Geometry: final body of the model. Coordinates: model frame, mm. Face numbers are marked on the shaded views. A direction names the side the tool comes from. Coordinates: 2 decimals unless noted, no trailing zeros. Write each loop counter-clockwise with the first axis right and the second up, starting at its lowest first coordinate (ties: lowest second). Pieces come first, ordered by that corner, then holes. Notation, with made-up numbers: (31.25, 79.5) -> (50.25, 79.5) arc R21 ccw to (50.25, 101.5) -> close; hole circle Ø10 at (48.5, 52). An arc over 180 degrees is marked (long way). One line per item, written item: value.
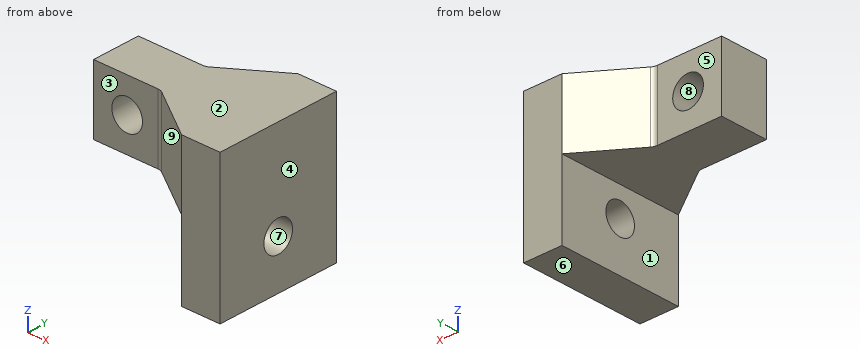
Autodesk Inventor part; units mm, degrees
ref_plane "YZ Plane" through (0, 0, 0) normal (1, 0, 0) x (0, 1, 0)
ref_plane "XZ Plane" through (0, 0, 0) normal (0, 1, 0) x (-1, 0, 0)
ref_plane "XY Plane" through (0, 0, 0) normal (0, 0, 1) x (1, 0, 0)
sketch "Sketch1" plane through (0, 0, 0) normal (1, 0, 0) x (0, 1, 0)
  circle A0 centre (0, 0) radius 1.6
  line L0 (0, 0) -> (0, -66.3)
  circle A1 centre (0, -66.3) radius 1.6
  line L1 (0, 0) -> (3.5, 0)
  line L2 (3.5, 0) -> (3.5, 3.5)
  line L3 (3.5, 3.5) -> (-3.5, 3.5)
  line L4 (-3.5, 3.5) -> (-3.5, -3.5)
  line L5 (-3.5, -3.5) -> (3.5, -3.5)
  line L6 (3.5, -3.5) -> (3.5, 0)
  line L7 (0, -66.3) -> (3.5, -66.3)
  line L8 (3.5, -66.3) -> (3.5, -62.8)
  line L9 (3.5, -62.8) -> (-3.5, -62.8)
  line L10 (-3.5, -62.8) -> (-3.5, -69.8)
  line L11 (-3.5, -69.8) -> (3.5, -69.8)
  line L12 (3.5, -69.8) -> (3.5, -66.3)
  line L13 (3.5, 3.5) -> (3.5, 6.5)
  line L14 (3.5, 6.5) -> (-3.5, 6.5)
  line L15 (-3.5, 6.5) -> (-3.5, 3.5)
  line L16 (3.5, -69.8) -> (3.5, -72.8)
  line L17 (3.5, -72.8) -> (-3.5, -72.8)
  line L18 (-3.5, -72.8) -> (-3.5, -69.8)
  dimension "d0" = 3.2
  dimension "d1" = 66.3
  dimension "d2" = 3.2
  dimension "d3" = 3.5
  dimension "d4" = 3.5
  dimension "d5" = 7
  dimension "d6" = 7
  dimension "d7" = 3.5
  dimension "d8" = 3.5
  dimension "d9" = 7
  dimension "d10" = 7
  dimension "d11" = 3
  dimension "d12" = 3
extrude "Extrusion1" add sketch "Sketch1" along normal blind 3 contours L1 L6 L5 L0 A0 | A0 L0 L5 L4 L3 L2 L1 | L9 L8 L7 A1 L0 | L0 A1 L7 L12 L11 L10 L9 | L3 L15 L14 L13 | L11 L16 L17 L18
sketch "Sketch2" plane through (3, 0, 0) normal (1, 0, 0) x (0, 0, -1)
  line L0 (-6.5, 3.5) -> (-6.5, -3.5)
  line L1 (-6.5, -3.5) -> (3.5, -3.5)
  line L2 (3.5, -3.5) -> (3.5, 3.5)
  line L3 (3.5, 3.5) -> (-6.5, 3.5)
  circle A0 centre (0, 0) radius 1.6
  line L4 (62.8, -3.5) -> (72.8, -3.5)
  line L5 (72.8, -3.5) -> (72.8, 3.5)
  line L6 (72.8, 3.5) -> (62.8, 3.5)
  line L7 (62.8, 3.5) -> (62.8, -3.5)
  circle A1 centre (66.3, 0) radius 1.6
  line L8 (-6.5, 3.5) -> (-6.5, -3.5)
  line L9 (-6.5, 3.5) -> (-2.5, 3.5)
  line L10 (3.5, 3.5) -> (-6.5, 3.5)
  line L11 (-2.5, 3.5) -> (-2.5, -3.5)
  line L12 (-6.5, -3.5) -> (3.5, -3.5)
  line L13 (-2.5, -3.5) -> (-6.5, -3.5)
  line L14 (72.8, 3.5) -> (68.8, 3.5)
  line L15 (72.8, 3.5) -> (62.8, 3.5)
  line L16 (68.8, 3.5) -> (68.8, -3.5)
  line L17 (62.8, -3.5) -> (72.8, -3.5)
  line L18 (72.8, -3.5) -> (68.8, -3.5)
  dimension "d15" = 4
  dimension "d16" = 4
extrude "Extrusion2" add sketch "Sketch2" along normal blind 10 contours L3 L11 L1 L0 | L16 L6 L5 L4
sketch "Sketch3" plane through (0, 0, 0) normal (-1, 0, 0) x (0, 0, 1)
  line L0 (6.5, 3.5) -> (6.5, -3.5)
  line L1 (-3.5, 3.5) -> (6.5, 3.5)
  line L2 (-3.5, -3.5) -> (-3.5, 3.5)
  line L3 (6.5, -3.5) -> (-3.5, -3.5)
  circle A0 centre (0, 0) radius 1.6
extrude "Extrusion3" cut sketch "Sketch3" against normal through all
sketch "Sketch4" plane through (0, -3.5, -72.8) normal (0, -1, 0) x (1, 0, 0)
  line L0 (0, 10) -> (0, 0)
  line L1 (0, 0) -> (13, 0)
  line L2 (13, 4) -> (13, 0)
  line L3 (3, 4) -> (13, 4)
  line L4 (3, 10) -> (3, 4)
  line L5 (0, 10) -> (3, 10)
  point P0 (0, 72.8)
extrude "Extrusion4" add sketch "Sketch4" along normal blind 3
sketch "Sketch5" plane through (0, 3.5, -62.8) normal (0, 1, 0) x (1, 0, 0)
  line L0 (0, 10) -> (0, 0)
  line L1 (0, 0) -> (3, 0)
  line L2 (3, 6) -> (3, 0)
  line L3 (3, 6) -> (13, 6)
  line L4 (13, 10) -> (13, 6)
  line L5 (0, 10) -> (13, 10)
  point P0 (0, -62.8)
extrude "Extrusion5" add sketch "Sketch5" along normal blind 3
sketch "Sketch6" plane through (13, 0, 0) normal (1, 0, 0) x (0, 0, -1)
  line L0 (68.8, -6.5) -> (68.8, 6.5)
  line L1 (72.8, -6.5) -> (68.8, -6.5)
  line L2 (72.8, 6.5) -> (72.8, -6.5)
  line L3 (68.8, 6.5) -> (72.8, 6.5)
  point P0 (0, 0)
extrude "Extrusion6" cut sketch "Sketch6" against normal blind 2
sketch "Sketch7" plane through (0, -6.5, -72.8) normal (0, 0, -1) x (-1, 0, 0)
  line L0 (0, 0) -> (-11, 0)
  line L1 (-11, 0) -> (-7, 0)
  line L2 (-7, 0) -> (-7, 13.1195)
  line L3 (-3, 0) -> (-3, 13)
  line L4 (-11, 13) -> (-11, 0)
  line L5 (0, 0) -> (-11, 0)
  line L6 (0, 13) -> (0, 0)
  line L7 (-11, 13) -> (0, 13)
  point P0 (0, 6.5)
  point P1 (-7, 13)
  dimension "d27" = 4
extrude "Extrusion7" add sketch "Sketch7" along normal blind 6 contours L0 L4 L7 L2
sketch "Sketch8" plane through (7, -6.5, -72.8) normal (-1, 0, 0) x (0, 0, 1)
  line L0 (0, 13) -> (0, 0)
  line L1 (0, 13) -> (-6, 13)
  line L2 (-6, 0) -> (-6, 13)
  line L3 (0, 0) -> (-6, 0)
  line L4 (-6, 13) -> (-6, 0)
  line L5 (-6, 0) -> (-6, 6.5)
  line L6 (-6, 6.5) -> (-3, 6.5)
  circle A0 centre (-3, 6.5) radius 1.6
  point P0 (72.8, 6.5)
  dimension "d30" = 6.5
  dimension "d31" = 3
  dimension "d32" = 3.2
extrude "Extrusion8" cut sketch "Sketch8" against normal blind 6 contours A0
sketch "Sketch9" plane through (3, 0, 0) normal (1, 0, 0) x (0, 0, -1)
  circle A0 centre (66.3, 0) radius 1.6
  line L0 (68.8, -6.5) -> (68.8, 6.5)
  line L1 (62.8, 6.5) -> (68.8, 6.5)
  line L2 (62.8, -6.5) -> (62.8, 6.5)
  line L3 (68.8, -6.5) -> (62.8, -6.5)
  point P0 (0, 0)
extrude "Extrusion9" cut sketch "Sketch9" against normal blind 6
sketch "Sketch10" plane through (0, 0, 0) normal (-1, 0, 0) x (0, 0, 1)
  line L0 (-68.8, -6.5) -> (-68.8, 6.5)
  line L1 (-72.8, 6.5) -> (-68.8, 6.5)
  line L2 (-72.8, 6.5) -> (-72.8, -6.5)
  line L3 (-68.8, -6.5) -> (-72.8, -6.5)
  point P0 (0, 0)
extrude "Extrusion10" add sketch "Sketch10" along normal blind 5.9
sketch "Sketch11" plane through (7, -6.5, -72.8) normal (0, 0, -1) x (-1, 0, 0)
  line L0 (0, 13) -> (0, 0)
  line L1 (0, 0) -> (12.9, 0)
  line L2 (12.9, 13) -> (12.9, 0)
  line L3 (0, 13) -> (12.9, 13)
  line L4 (-4, 0) -> (12.9, 0)
  line L5 (12.9, 0) -> (12.9, 5)
  line L6 (12.9, 13) -> (12.9, 0)
  line L7 (12.9, 5) -> (12.9, 8)
  line L8 (12.9, 8) -> (6.9, 8)
  line L9 (0, 0) -> (0, 13)
  line L10 (6.9, 8) -> (0, 13)
  line L11 (12.9, 5) -> (6.9, 5)
  line L12 (-4, 0) -> (0, 0)
  line L13 (6.9, 5) -> (0, 0)
  point P0 (7, 6.5)
  dimension "d39" = 5
  dimension "d40" = 3
  dimension "d41" = 6
extrude "Extrusion11" cut sketch "Sketch11" against normal blind 5.9 contours L3 L2 L8 L10 | L13 L11 L2 L1
sketch "Sketch12" plane through (11, -6.5, -68.8) normal (0, 0, 1) x (1, 0, 0)
  line L0 (-10.9, 5) -> (-4, 0)
  line L1 (0, 0) -> (-4, 0)
  line L2 (0, 0) -> (0, 13)
  line L3 (0, 13) -> (-4, 13)
  line L4 (-4, 13) -> (-10.9, 8)
  line L5 (-10.9, 8) -> (-16.9, 8)
  line L6 (-16.9, 5) -> (-16.9, 8)
  line L7 (-16.9, 5) -> (-10.9, 5)
  point P0 (-11, 6.5)
extrude "Extrusion12" add sketch "Sketch12" along normal blind 3
sketch "Sketch13" plane through (-5.9, -1.5, -72.8) normal (0, -1, 0) x (1, 0, 0)
  line L0 (6, 0) -> (0, 0)
  line L1 (0, 0) -> (0, 3.5)
  line L2 (0, 0) -> (0, 7)
  line L3 (0, 0) -> (0, 7)
  line L4 (6, 0) -> (0, 0)
  line L5 (6, 0) -> (6, 7)
  line L6 (0, 7) -> (6, 7)
  line L7 (0, 3.5) -> (3.5, 3.5)
  circle A0 centre (3.5, 3.5) radius 1.6
  point P0 (5.9, 72.8)
  dimension "d46" = 3.5
  dimension "d47" = 3.5
  dimension "d48" = 3.2
extrude "Extrusion13" cut sketch "Sketch13" against normal through all contours A0
sketch "Sketch14" plane through (11, -6.5, -65.8) normal (0, 0, 1) x (1, 0, 0)
  line L0 (-10.9, 5) -> (-4, 0)
  line L1 (-4, 0) -> (0, 0)
  line L2 (0, 0) -> (0, 13)
  line L3 (0, 13) -> (-4, 13)
  line L4 (-4, 13) -> (-10.9, 8)
  line L5 (-10.9, 8) -> (-16.9, 8)
  line L6 (-16.9, 8) -> (-16.9, 5)
  line L7 (-16.9, 5) -> (-10.9, 5)
  line L8 (-4, 13) -> (-10.9, 8)
  line L9 (-10.9, 8) -> (-9.9, 8)
  line L10 (-9.9, 8) -> (-4, 13)
  line L11 (-4, 0) -> (-10.9, 5)
  line L12 (-10.9, 5) -> (-9.9, 5)
  line L13 (-9.9, 5) -> (-4, 0)
  point P0 (-11, 6.5)
  dimension "d52" = 1
extrude "Extrusion14" cut sketch "Sketch14" against normal blind 10 contours L12 L13 L0 | L4 L10 L9
sketch "Sketch15" plane through (0, -6.5, -78.8) normal (0, 0, -1) x (-1, 0, 0)
  line L0 (-11, 0) -> (-7, 0)
  line L1 (-7, 0) -> (-7, 13)
  line L2 (-7, 13) -> (-11, 13)
  line L3 (-11, 13) -> (-11, 0)
  point P0 (0, 6.5)
extrude "Extrusion15" add sketch "Sketch15" along normal blind 2
sketch "Sketch16" plane through (-5.9, 1.5, -65.8) normal (0, 1, 0) x (1, 0, 0)
  circle A0 centre (3.5, 3.5) radius 1.6
  line L0 (0, 7) -> (7, 7)
  line L1 (0, 0) -> (0, 7)
  line L2 (7, 0) -> (0, 0)
  line L3 (7, 0) -> (7, 7)
  point P0 (5.9, -65.8)
extrude "Extrusion16" add sketch "Sketch16" along normal blind 1
sketch "Sketch17" plane through (-5.9, -1.5, -72.8) normal (0, -1, 0) x (1, 0, 0)
  circle A0 centre (3.5, 3.5) radius 1.6
  line L0 (0, 0) -> (0, 7)
  line L1 (7, 0) -> (0, 0)
  line L2 (7, 7) -> (7, 0)
  line L3 (0, 7) -> (7, 7)
  point P0 (5.9, 72.8)
extrude "Extrusion17" add sketch "Sketch17" along normal blind 1
sketch "Sketch18" plane through (7, -6.5, -72.8) normal (0, 0, -1) x (-1, 0, 0)
  line L0 (12.9, 9) -> (12.9, 4)
  line L1 (5.9, 9) -> (12.9, 9)
  line L2 (5.9, 8) -> (5.9, 9)
  line L3 (5.9, 8) -> (0, 13)
  line L4 (0, 13) -> (0, 0)
  line L5 (0, 0) -> (5.9, 5)
  line L6 (5.9, 5) -> (5.9, 4)
  line L7 (12.9, 4) -> (5.9, 4)
  line L8 (5.9, 4) -> (0, 0)
  line L9 (12.9, 9) -> (5.9, 9)
  line L10 (0, 13) -> (5.9, 8)
  line L11 (5.9, 9) -> (0, 13)
  point P0 (7, 6.5)
extrude "Extrusion18" add sketch "Sketch18" against normal blind 7 contours L2 L3 L11 | L8 L5 L6
fillet "Fillet3" radius 1 2 edges at (1.1, -2.5, -69.3) (1.1, 2.5, -69.3)
properties part number "base_servos"
(1) Pull-direction query (Z, two-part tool) for the marked faces 6, 7, 8 and 9; classes: released by +Z, released by -Z, zero draft, split by the parting line, or undercut.
Responses:
face 6: released by -Z
face 7: undercut
face 8: undercut
face 9: zero draft
(2) Line query: line 1 (X direction, y = 1.45, z = -69.3); line 2 (Y direction, x = 9.1, z = -75.8); line 3 (Z direction, x = -2.4, y = 0.4). Output: solid intervals per line, ascending. Write a range as [from, to].
Responses:
line 1: x = [-5.9, -4], [-0.8, 11]
line 2: y = [-6.5, -1.6], [1.6, 6.5]
line 3: z = [-72.8, -70.9], [-67.7, -65.8]
(3) Section B-B (y = 0). Return the cut outline in (x, z).
Responses:
outline: (-5.9, -72.8) -> (7, -72.8) -> (7, -74.2) -> (11, -74.2) -> (11, -65.8) -> (-5.9, -65.8) -> close; (7, -80.8) -> (11, -80.8) -> (11, -77.4) -> (7, -77.4) -> close; hole circle Ø3.2 at (-2.4, -69.3)
(4) Section C-C (x = -2.4). Return the cut outline in (y, z).
Responses:
outline: (-2.5, -72.8) -> (2.5, -72.8) -> (2.5, -70.9) -> (-2.5, -70.9) -> close; (-2.5, -67.7) -> (2.5, -67.7) -> (2.5, -65.8) -> (-2.5, -65.8) -> close
(5) Reachability of the marked faces 1, 2, 3, 4 and 5 from +Z, -Z, +X, -X, +Y, -Y: full face, straight path, thin tool, end or side. Return the list, or none.
Responses:
face 1: -Z, -X, +Y, -Y
face 2: +Z, +X, -X, +Y, -Y
face 3: +Z, -Z, -X, -Y
face 4: +Z, -Z, +X, +Y, -Y
face 5: +Z, -Z, -X, +Y
(6) Section D-D (x = 7.75). Return the cut outline in (y, z).
Responses:
outline: (-6.5, -80.8) -> (6.5, -80.8) -> (6.5, -65.8) -> (-6.5, -65.8) -> close; hole circle Ø3.2 at (0, -75.8)
(7) Section A-A (z = -69.3). Return the cut outline in (x, y).
Responses:
outline: (-5.9, -2.5) -> (-4, -2.5) -> (-4, 2.5) -> (-5.9, 2.5) -> close; (-0.8, -2.5) -> (0.79, -2.5) arc R1 cw to (1.35, -2.67) -> (7, -6.5) -> (11, -6.5) -> (11, 6.5) -> (7, 6.5) -> (1.35, 2.67) arc R1 cw to (0.79, 2.5) -> (-0.8, 2.5) -> close
(8) First-contact query: pin 1 (3 mm diameter, centred on x = 6, y = -3, fed in from -Z); pin 2 (5.5 mm diameter, centred on x = -1.5, z = -67.5, fed in from +Y); pin 3 (2 mm diameter, centred on x = -2, z = -70.5, fed in from -Y); pin 4 (6.5 mm diameter, centred on x = -2, y = 0.5, fed in from -Z). Flat tips, straight axial feed; report the tip coordinate or a pass-through.
Responses:
pin 1: stops at z = -80.8
pin 2: stops at y = 2.61
pin 3: stops at y = -2.5
pin 4: stops at z = -72.8
